from build123d import *

# Parameters (mm, degrees)
BOSS_EXTRUDE1_DEPTH = 3.175
FILLET1_R           = 7
FILLET2_R           = 5
SKETCH2_R           = 2.38125
CUT_EXTRUDE1_DEPTH  = 51.309846203
LPATTERN1_COUNT     = 3
LPATTERN1_PITCH     = 12.5


with BuildPart() as part:
    # Sketch1 → Boss-Extrude1 (new body)
    with BuildSketch(Plane.XY):
        with BuildLine():
            Line((-11.618950039, 11), (-36, 11))
            Line((-36, 11), (-36, -24))
            ThreePointArc((-36, -24), (-25, -35), (-14, -24))
            Line((-14, -24), (-14, -11))
            Line((-14, -11), (-11.618950039, -11))
            ThreePointArc((-11.618950039, -11), (16, 0), (-11.618950039, 11))
        make_face()
    extrude(amount=BOSS_EXTRUDE1_DEPTH)

    # Fillet1
    fillet1_edges = [part.edges().sort_by_distance(p)[0] for p in [
        (-36, 11, 1.5875),
    ]]
    fillet(fillet1_edges, radius=FILLET1_R)

    # Fillet2
    # the kernel refuses this fillet: 5 mm, written as the material it adds along each edge
    with BuildSketch(Plane(origin=(-14, -11, 0), x_dir=(1, 0, 0), z_dir=(0, 0, 1))) as fillet2_piece_1:
        with BuildLine():
            CenterArc((5, -4.259237102), FILLET2_R, 121.586822832, 58.413177168)
            Line((0, -4.259237102), (-0.1, -4.259237102))
            Line((-0.1, -4.259237102), (-0.1, 0))
            Line((-0.1, 0), (0, 0.1))
            ThreePointArc((0, 0.1), (1.190524981, 0.1), (2.328670961, 0.085184742))
            Line((2.328670961, 0.085184742), (2.381049961, 0))
        make_face()
    extrude(amount=3.175)

    # Sketch2 → Cut-Extrude1 (cut, through all)
    with BuildSketch(Plane.XY.offset(3.175)):
        Circle(SKETCH2_R)
    cut_extrude1 = extrude(amount=-CUT_EXTRUDE1_DEPTH, mode=Mode.SUBTRACT)

    # LPattern1: Cut-Extrude1 ×3
    with Locations(*[(-i * LPATTERN1_PITCH, 0, 0) for i in range(1, LPATTERN1_COUNT)]):
        add(cut_extrude1, mode=Mode.SUBTRACT)


solid = part.part
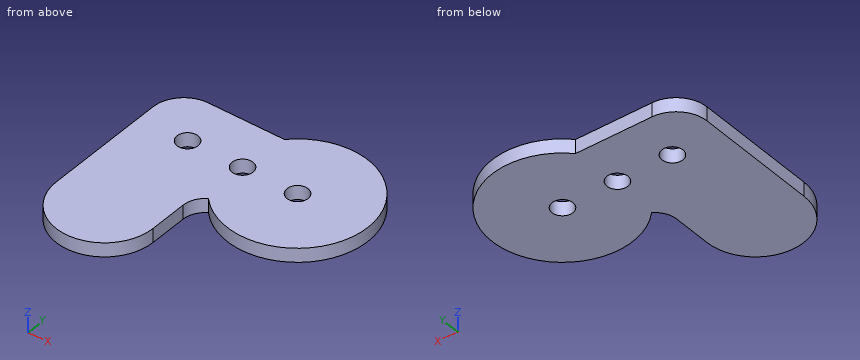
Verification items for the finished model (mm, model axes). Round coordinates to 2 decimals unless told otherwise and drop trailing zeros. Order: outer loops, then holes, each group sorted by start corner. A loop starts at its lowest first (then second) coordinate and runs counter-clockwise, first axis right, second up.
1. Section check D-D on y = 1. Record the cut outline in (x, z) (3 decimals).
Final values:
outline: (-36, 0) - (-27.161, 0) - (-27.161, 3.175) - (-36, 3.175) - close; (-22.839, 0) - (-14.661, 0) - (-14.661, 3.175) - (-22.839, 3.175) - close; (-10.339, 0) - (-2.161, 0) - (-2.161, 3.175) - (-10.339, 3.175) - close; (2.161, 0) - (15.969, 0) - (15.969, 3.175) - (2.161, 3.175) - close
2. Section check C-C on x = -25. Record the cut outline in (y, z) (3 decimals).
Final values:
outline: (-35, 0) - (-2.381, 0) - (-2.381, 3.175) - (-35, 3.175) - close; (2.381, 0) - (11, 0) - (11, 3.175) - (2.381, 3.175) - close
3. Thickness scan on L1, parallel to Y at x = 0, z = 1.25; L2, parallel to X at y = -2, z = 1.7; L3, parallel to Y at x = -23.5, z = 0.2. Record the ranges inside material, lowest first.
Final values:
L1: y = -16 to -2.38, 2.38 to 16
L2: x = -36 to -26.29, -23.71 to -13.79, -11.21 to -1.29, 1.29 to 15.87
L3: y = -34.9 to -1.85, 1.85 to 11
4. Go/stop test with flat-tipped pins: P1, Ø12, axis at x = -25.5, y = 9, coming from the -Z side; P2, Ø1.5, axis at x = -29, z = 1.5, coming from the -Y side; P3, Ø1.6, axis at x = -19, z = 1, coming from the +Y side. Record where each tip stops, or that it passes through.
Final values:
P1: stops at z = 0
P2: stops at y = -34.51
P3: stops at y = 11
5. Section check A-A on x = 0. Record the cut outline in (y, z) (3 decimals), then the cut area to 3 significant figures.
Final values:
outline: (-16, 0) - (-2.381, 0) - (-2.381, 3.175) - (-16, 3.175) - close; (2.381, 0) - (16, 0) - (16, 3.175) - (2.381, 3.175) - close
area: 86.5 mm2
6. Section check B-B on z = 0.8. Record the cut outline in (x, y).
Final values:
outline: (-36, -24) arc R11 ccw to (-14, -24) - (-14, -15.26) arc R5 cw to (-11.62, -11) arc R16 ccw (long way) to (-11.62, 11) - (-29, 11) arc R7 ccw to (-36, 4) - close; hole circle Ø4.76 at (-25, 0); hole circle Ø4.76 at (-12.5, 0); hole circle Ø4.76 at (0, 0)
